The drawing under review shows one solid part. Ordinate dimensions are in mm from its lowest x, y, z. Coordinates: 2 decimals unless noted, no trailing zeros. Order: outer loops, then holes, each group sorted by start corner. A loop starts at its lowest first (then second) coordinate and runs counter-clockwise, first axis right, second up. Notation, with made-up numbers: (55, -16) -> (109, -16) arc R29 cw to (109, 15) -> close; hole circle Ø5 at (-34, 55). An arc over 180 degrees is marked (long way). Use one line per item in the form item = value.
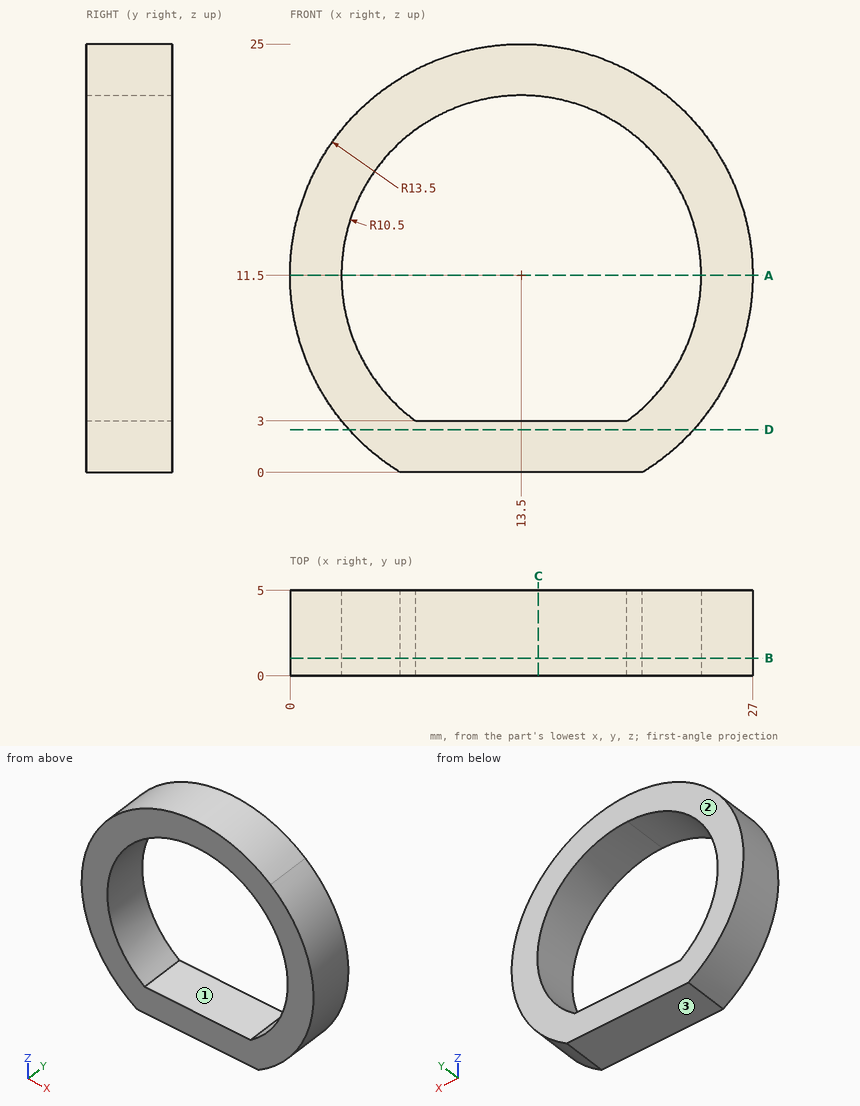
Item 1: Draft analysis for pull direction Z (two halves, no side actions). For the marked faces 1, 2 and 3, state which applies: released by +Z, released by -Z, zero draft, split by the parting line, or undercut.
Results found:
face_1 = undercut
face_2 = zero draft
face_3 = released by -Z
Item 2: We need section B-B (y = 1.05). Write out the cut boundary in (x, z), plus the area to 3 significant figures.
Results found:
outline = (6.43, 0) -> (20.57, 0) arc R13.5 ccw (long way) to start; hole (7.34, 3) -> (19.66, 3) arc R10.5 ccw (long way) to start
area = 224 mm²
Item 3: To check wall thickness, follow L1, parallel to X at y = 1.45, z = 11.25; L2, parallel to Z at x = 13.25, y = 1.85; L3, parallel to X at y = 1.7, z = 3.25. State the ranges of each line that lie inside material, in increasing order. Write a range as from..to.
Results found:
L1 = 0..3, 24..27
L2 = 0..3, 22..25
L3 = 2.81..7, 20..24.19
Item 4: We need section C-C (x = 14.5). Write out the cut boundary in (y, z), plus the area to 3 significant figures.
Results found:
outline = (0, 0) -> (5, 0) -> (5, 3) -> (0, 3) -> close; (0, 21.95) -> (5, 21.95) -> (5, 24.96) -> (0, 24.96) -> close
area = 30.1 mm²
Item 5: We need section D-D (z = 2.5). Write out the cut boundary in (x, y).
Results found:
outline = (3.44, 0) -> (23.56, 0) -> (23.56, 5) -> (3.44, 5) -> close
Item 6: Clearance check with flat-ended pins moving along their axes: pin 1 (2 mm diameter, centred on x = 21, y = 1.5, fed in from +Z); pin 2 (1 mm diameter, centred on y = 3, z = 15, fed in from -X). State where each tip first meets the part, or that it passes through.
Results found:
pin_1 = 23.33
pin_2 = 0.34
Item 7: We need section A-A (z = 11.5). Write out the cut boundary in (x, y).
Results found:
outline = (0, 0) -> (3, 0) -> (3, 5) -> (0, 5) -> close; (24, 0) -> (27, 0) -> (27, 5) -> (24, 5) -> close
